Check sheet for the drawn part. Datum: minimum x, y, z corner. Units: mm. Give positions to 0.01 mm unless a question says otherwise; leave off trailing zeros. Order: outer loops, then holes, each group sorted by start corner. A loop starts at its lowest first (then second) coordinate and runs counter-clockwise, first axis right, second up. Notation, with made-up numbers: (-26, 25) -> (13, 25) arc R19 cw to (13, 39) -> close; hole circle Ø4 at (89.25, -11.5). An arc over 180 degrees is marked (long way). Answer in a Markdown table with one row per item. Add a question column.
(1) Cross-section at D-D (x = 49.5). Record the cut outline in (y, z) (1 decimal).
(2) Cross-section at B-B (z = 2). Record the cut outline in (x, y).
(3) Cross-section at A-A (x = 35). Record the cut outline in (y, z).
(4) Cross-section at C-C (y = 46). Record the cut outline in (x, z).
(5) Thickness scan on L1, parallel to Y at x = 35, z = 2.4; L2, parallel to Y at x = 58.5, z = 1.3; L3, parallel to Y at x = 22.5, z = 0.6. Record the ranges inside material, lowest first. Write a range as [from, to].
(6) Go/stop test with flat-tipped pins: pin 1 (1 mm diameter, centred on x = 31, z = 1.5, fed in from +Y); pin 2 (1 mm diameter, centred on y = 55, z = 1, fed in from -X) (1 decimal); pin 3 (1.5 mm diameter, centred on y = 49.5, z = 0.5, fed in from -X). Record where each tip stops, or that it passes through.
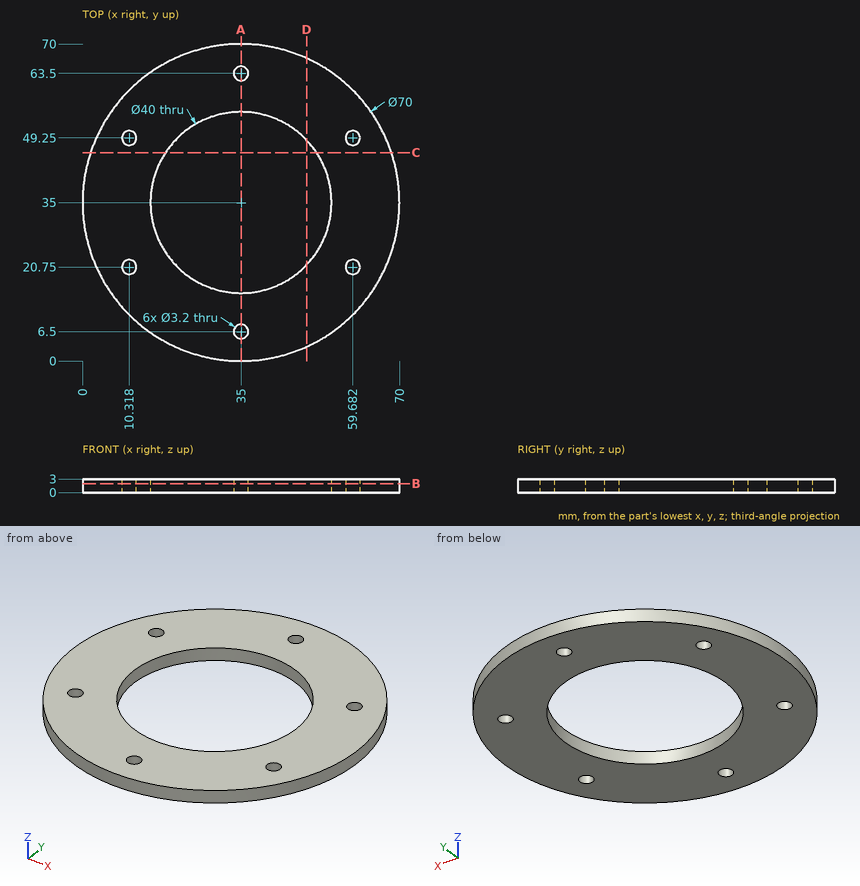
Answer below:
| question | item | result |
|---|---|---|
| 1 | outline | (3.1, 0) -> (21.2, 0) -> (21.2, 3) -> (3.1, 3) -> close; (48.8, 0) -> (66.9, 0) -> (66.9, 3) -> (48.8, 3) -> close |
| 2 | outline | circle Ø70 at (35, 35); hole circle Ø3.2 at (10.32, 20.75); hole circle Ø3.2 at (10.32, 49.25); hole circle Ø40 at (35, 35); hole circle Ø3.2 at (35, 6.5); hole circle Ø3.2 at (35, 63.5); hole circle Ø3.2 at (59.68, 20.75); hole circle Ø3.2 at (59.68, 49.25) |
| 3 | outline | (0, 0) -> (4.9, 0) -> (4.9, 3) -> (0, 3) -> close; (8.1, 0) -> (15, 0) -> (15, 3) -> (8.1, 3) -> close; (55, 0) -> (61.9, 0) -> (61.9, 3) -> (55, 3) -> close; (65.1, 0) -> (70, 0) -> (70, 3) -> (65.1, 3) -> close |
| 4 | outline | (1.77, 0) -> (18.3, 0) -> (18.3, 3) -> (1.77, 3) -> close; (51.7, 0) -> (68.23, 0) -> (68.23, 3) -> (51.7, 3) -> close |
| 5 | L1 | y = [0, 4.9], [8.1, 15], [55, 61.9], [65.1, 70] |
| 5 | L2 | y = [9.06, 19.67], [21.83, 48.17], [50.33, 60.94] |
| 5 | L3 | y = [2.31, 19.39], [50.61, 67.69] |
| 6 | pin 1 | stops at y = 69.82 |
| 6 | pin 2 | stops at x = 5.9 |
| 6 | pin 3 | stops at x = 2.81 |
